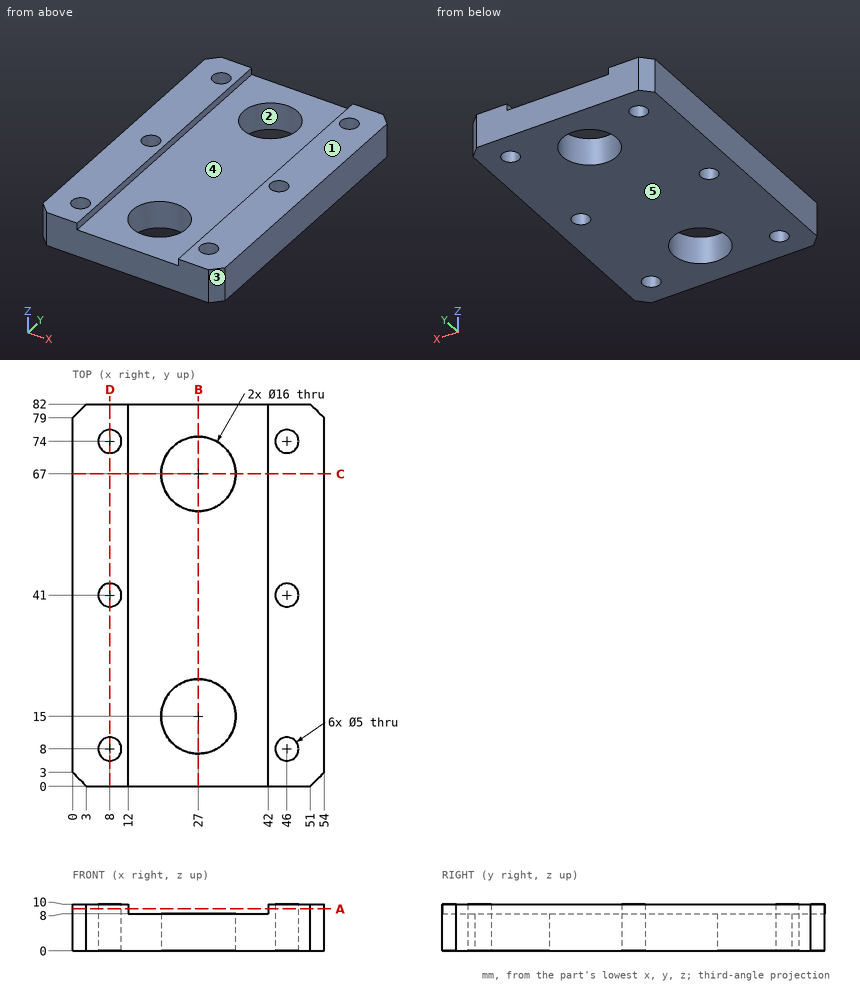
Check sheet for the drawn part. Datum: minimum x, y, z corner. Units: mm. A direction names the side the tool comes from. Round coordinates to 2 decimals unless told otherwise and drop trailing zeros. Write each loop counter-clockwise with the first axis right and the second up, starting at its lowest first coordinate (ties: lowest second). Pieces come first, ordered by that corner, then holes. Notation, with made-up numbers: (-4, -9.5) - (52, -9.5) arc R32 cw to (52, 23.5) - close; hole circle Ø9 at (73, 68). An arc over 180 degrees is marked (long way). Write each question's results on one line, items separated by ' | '.
(1) Sectioned sample at A-A, the plane z = 9. Enter the section's corners in (x, y).
Computed:
outline: (0, 3) - (3, 0) - (12, 0) - (12, 82) - (3, 82) - (0, 79) - close; (42, 0) - (51, 0) - (54, 3) - (54, 79) - (51, 82) - (42, 82) - close; hole circle Ø5 at (8, 8); hole circle Ø5 at (8, 41); hole circle Ø5 at (8, 74); hole circle Ø5 at (46, 8); hole circle Ø5 at (46, 41); hole circle Ø5 at (46, 74)
(2) Thickness scan on probe 1 along Y at (x, z) = (46, 4); probe 2 along Y at (x, z) = (27, 4.75); probe 3 along X at (y, z) = (15, 4). Record the ranges inside material, lowest first. Write a range as from..to.
Computed:
probe 1: y = 0..5.5, 10.5..38.5, 43.5..71.5, 76.5..82 | probe 2: y = 0..7, 23..59, 75..82 | probe 3: x = 0..19, 35..54
(3) Sectioned sample at B-B, the plane x = 27. Enter the section's corners in (y, z), plus the area to 3 significant figures.
Computed:
outline: (0, 0) - (7, 0) - (7, 8) - (0, 8) - close; (23, 0) - (59, 0) - (59, 8) - (23, 8) - close; (75, 0) - (82, 0) - (82, 8) - (75, 8) - close | area: 400 mm^2
(4) Draft check along X on the marked faces 1, 2 and 3. Enter one of: pulls with the +X half, pulls with the -X half, needs draft (parallel to the pull), parting line crosses it, or undercut.
Computed:
face 1: needs draft | face 2: undercut | face 3: pulls with the +X half
(5) Sectioned sample at D-D, the plane x = 8. Enter the section's corners in (y, z), plus the area to 3 significant figures.
Computed:
outline: (0, 0) - (5.5, 0) - (5.5, 10) - (0, 10) - close; (10.5, 0) - (38.5, 0) - (38.5, 10) - (10.5, 10) - close; (43.5, 0) - (71.5, 0) - (71.5, 10) - (43.5, 10) - close; (76.5, 0) - (82, 0) - (82, 10) - (76.5, 10) - close | area: 670 mm^2
(6) Sectioned sample at C-C, the plane y = 67. Enter the section's corners in (x, z).
Computed:
outline: (0, 0) - (19, 0) - (19, 8) - (12, 8) - (12, 10) - (0, 10) - close; (35, 0) - (54, 0) - (54, 10) - (42, 10) - (42, 8) - (35, 8) - close
(7) Depth check by flat-ended pin: pin 1 Ø21 at (x, y) = (27, 67) entering from +Z. Enter the tip coordinate at first touch or a pass-through.
Computed:
pin 1: stops at z = 8
(8) Set-up check for the marked faces 4 and 5: record each of +Z, -Z, +X, -X, +Y, -Y from which the full face is reachable in a straight line by a thin tool's end or side.
Computed:
face 4: +Z, +Y, -Y | face 5: -Z, +X, -X, +Y, -Y
